The listing builds one solid part. Answer for the finished solid, in the listing's coordinates (mm). Give positions to 0.01 mm unless a question says otherwise; leave off trailing zeros. Write each loop counter-clockwise with the first axis right and the second up, starting at its lowest first coordinate (ties: lowest second). Pieces come first, ordered by that corner, then holes. Notation, with made-up numbers: (53, 0) - (94, 0) arc R15 cw to (94, 17) - close; hole circle Ø9 at (-16.5, -8.75). An arc over 180 degrees is marked (long way). Write each question's results on one line, items separated by ' | '. Start each with the question number.
Q1. Section B-B (x = 163) is taken. Determine the outline of the cut face in (y, z), plus the area to 3 significant figures.
Q2. Section A-A (x = 34.5) is taken. Determine the outline of the cut face in (y, z).
Q3. Flat-ended cylindrical pins translate along their axes: pin 1 Ø4 at (x, y) = (0.54, -30.15) entering from -Z; pin 2 Ø1.2 at (y, z) = (6, 2) entering from +X; pin 3 Ø3 at (x, y) = (27.54, 35.7) entering from +Z; pin 4 Ø2 at (x, z) = (-0.5, 1.5) entering from -Y. Find the tip coordinate at first contact, or state that the pin passes through.
Q4. Section C-C (z = 2.9) is taken. State how many separate pieces and enclosed holes the cut face has, plus the area to 3 significant figures.
Q5. Find the intervals of material crossed by probe 1 along Y at (x, z) = (112.5, 0.6); probe 2 along Y at (x, z) = (50, 3); probe 3 along Y at (x, z) = (142, 1.7), in increasing order.
```python
from build123d import *

# Parameters (mm, degrees)
EXTRUDE_1_OUTLINE_R   = 1.5
EXTRUDE_1_OUTLINE_W   = 4.3
EXTRUDE_1_OUTLINE_H   = 8.3
EXTRUDE_1_OUTLINE_R_2 = 11.5
EXTRUDE_1_OUTLINE_R_3 = 7.04
EXTRUDE_1_DEPTH       = 4
SKETCH_2_W            = 44
SKETCH_2_H            = 44
CUT_EXTRUDE_1_DEPTH   = 4
SKETCH_3_R            = 2
CUT_EXTRUDE_2_DEPTH   = 4
SKETCH_4_W            = 10
SKETCH_4_H            = 47.093490756
EXTRUDE_2_DEPTH       = 4
SKETCH_7_R            = 2
CUT_EXTRUDE_3_DEPTH   = 4


# Read off the part's stored shape, not the designer's step: 凸台-拉伸1
with BuildPart() as part:
    # 凸台-拉伸1 outline → 凸台-拉伸1 (new body)
    with BuildSketch(Plane.XY):
        with BuildLine():
            Line((174.542857143, -46.295714286), (199.556073527, -38.70591431))
            Line((199.556073527, -38.70591431), (230.542857143, -31.145714286))
            ThreePointArc((230.542857143, -31.145714286), (261.542857143, -0.145714286), (230.542857143, 30.854285714))
            Line((230.542857143, 30.854285714), (199.542857143, 41.704285714))
            Line((199.542857143, 41.704285714), (18.542857143, 41.704285714))
            Line((18.542857143, 41.704285714), (18.542857143, 14.854285714))
            Line((18.542857143, 14.854285714), (9.542857143, 14.854285714))
            Line((9.542857143, 14.854285714), (9.542857143, 41.704285714))
            Line((9.542857143, 41.704285714), (-5.457142857, 41.704285714))
            Line((-5.457142857, 41.704285714), (-5.457142857, -38.295714286))
            Line((-5.457142857, -38.295714286), (2.692857143, -38.295714286))
            Line((2.692857143, -38.295714286), (34.542857143, -46.295714286))
            Line((34.542857143, -46.295714286), (174.542857143, -46.295714286))
        make_face()
        with Locations((0.542857143, -30.145714286)):
            Circle(EXTRUDE_1_OUTLINE_R, mode=Mode.SUBTRACT)
        with Locations((0.542857143, -15.145714286)):
            Rectangle(EXTRUDE_1_OUTLINE_W, EXTRUDE_1_OUTLINE_H, mode=Mode.SUBTRACT)
        with Locations((50.542857143, -14.145714286)):
            Circle(EXTRUDE_1_OUTLINE_R, mode=Mode.SUBTRACT)
        with Locations((0.542857143, -0.145714286)):
            Circle(EXTRUDE_1_OUTLINE_R, mode=Mode.SUBTRACT)
        with Locations((36.542857143, -0.145714286)):
            Circle(EXTRUDE_1_OUTLINE_R, mode=Mode.SUBTRACT)
        with Locations((50.542857143, -0.145714286)):
            Circle(EXTRUDE_1_OUTLINE_R_2, mode=Mode.SUBTRACT)
        with Locations((0.542857143, 14.854285714)):
            Rectangle(EXTRUDE_1_OUTLINE_W, EXTRUDE_1_OUTLINE_H, mode=Mode.SUBTRACT)
        with Locations((50.542857143, 13.854285714)):
            Circle(EXTRUDE_1_OUTLINE_R, mode=Mode.SUBTRACT)
        with Locations((64.542857143, -0.145714286)):
            Circle(EXTRUDE_1_OUTLINE_R, mode=Mode.SUBTRACT)
        with Locations((0.542857143, 29.854285714)):
            Circle(EXTRUDE_1_OUTLINE_R, mode=Mode.SUBTRACT)
        with Locations((230.542857143, -0.145714286)):
            Circle(EXTRUDE_1_OUTLINE_R_3, mode=Mode.SUBTRACT)
    extrude(amount=EXTRUDE_1_DEPTH)

    # 草图2 → 切除-拉伸1 (cut)
    with BuildSketch(Plane.XY.offset(4)):
        with Locations((50.542857143, -0.145714286)):
            Rectangle(SKETCH_2_W, SKETCH_2_H)
    extrude(amount=-CUT_EXTRUDE_1_DEPTH, mode=Mode.SUBTRACT)

    # 草图3 → 切除-拉伸2 (cut)
    with BuildSketch(Plane.XY.offset(4)):
        with Locations((27.542857143, 35.704285714)):
            Circle(SKETCH_3_R)
        with Locations((112.542857143, 35.704285714)):
            Circle(SKETCH_3_R)
        with Locations((197.542857143, 35.704285714)):
            Circle(SKETCH_3_R)
        with Locations((112.542857143, -34.295714286)):
            Circle(SKETCH_3_R)
        with Locations((197.542857143, -34.295714286)):
            Circle(SKETCH_3_R)
        with Locations((27.542857143, -34.295714286)):
            Circle(SKETCH_3_R)
        Polygon((187.542857143, -24.295714286), (140.41622539, -24.295714286), (187.542857143, 14.51445304), align=None)
        Polygon((122.542857143, 25.704285714), (169.669488896, 25.704285714), (122.542857143, -13.105881612), align=None)
        Polygon((82.542857143, 14.734304613), (102.542857143, 21.659304613), (102.542857143, -20.807070509), (82.542857143, -14.732070509), align=None)
    extrude(amount=-CUT_EXTRUDE_2_DEPTH, mode=Mode.SUBTRACT)

    # 草图4 → 凸台-拉伸2 (add)
    with BuildSketch(Plane.XY.offset(4)):
        with Locations((139.542857143, 15.704285714)):
            Rectangle(SKETCH_4_W, SKETCH_4_H)
    extrude(amount=-EXTRUDE_2_DEPTH)

    # 草图7 → 切除-拉伸3 (cut)
    with BuildSketch(Plane.XY.offset(4)):
        with Locations((190.542857143, -0.145714286)):
            Circle(SKETCH_7_R)
        with Locations((140.542857143, 16.354285714)):
            Circle(SKETCH_7_R)
        with Locations(Location((140.542857143, -16.645714286, 0), (0, 0, 180))):
            Circle(SKETCH_7_R)
        Polygon((10.655357143, -40.295714286), (194.316671838, -40.295714286), (206.19710926, -67.618852766), (10.655357143, -65.874099546), align=None)
    extrude(amount=-CUT_EXTRUDE_3_DEPTH, mode=Mode.SUBTRACT)


solid = part.part
```
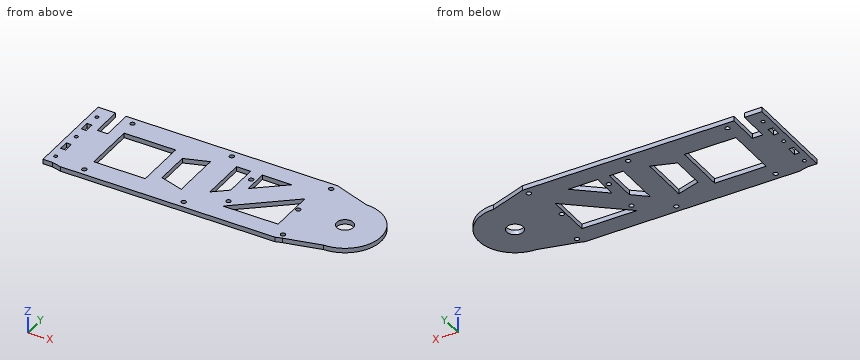
Answers below:
1) outline: (-40.3, 0) - (-24.3, 0) - (-24.3, 4) - (-40.3, 4) - close; (-5.7, 0) - (20.21, 0) - (20.21, 4) - (-5.7, 4) - close; (25.7, 0) - (41.7, 0) - (41.7, 4) - (25.7, 4) - close | area: 232 mm2
2) outline: (-40.3, 0) - (-22.15, 0) - (-22.15, 4) - (-40.3, 4) - close; (21.85, 0) - (41.7, 0) - (41.7, 4) - (21.85, 4) - close
3) pin 1: stops at z = 0 | pin 2: stops at x = 261.04 | pin 3: passes through | pin 4: stops at y = -38.3
4) separate pieces: 1 | enclosed holes: 20 | area: 15,700 mm2
5) probe 1: y = -40.3 to -36.3, -32.3 to 33.7, 37.7 to 41.7 | probe 2: y = -40.3 to -22.15, 21.85 to 41.7 | probe 3: y = -40.3 to -24.3, -22.99 to -18.02, -15.28 to 14.98, 17.72 to 41.7
